The model under review builds one solid part; all positions refer to its coordinate system, in mm. Face numbers are marked on the shaded views. Give positions to 0.01 mm unless a question says otherwise; leave off trailing zeros. Order: outer loops, then holes, each group sorted by start corner. A loop starts at its lowest first (then second) coordinate and runs counter-clockwise, first axis right, second up. Notation, with made-up numbers: (76, 69.25) - (132, 69.25) arc R19 cw to (132, 91.25) - close; hole circle Ø7 at (-3.75, 0.5). An arc over 180 degrees is marked (long way). Use CSV: the item, a comma, the result in double quotes. Start each with the question number.
1. Take a section at A-A, the plane z = -17.68. State the section outline as (x, y) points.
2. Take a section at B-B, the plane x = 0. State the section outline as (y, z) points (3 decimals), then the cut area to 3 significant figures.
3. For pin 1 (3 mm diameter, centred on x = 40.5, y = 1, fed in from -Z), flat-tipped, find the tip position at first contact; note if it passes through.
4. To check wall thickness, follow line 1 (X direction, y = 1.6, z = -35.36) (3 decimals); line 2 (Z direction, x = 0, y = 2.2) (3 decimals); line 3 (Z direction, x = 17.68, y = 2.3). State the ranges of each line that lie inside material, in increasing order. Write a range as [from, to].
5. Take a section at C-C, the plane y = 2.95. State the section outline as (x, z) points (3 decimals), then the cut area to 3 significant figures.
6. Draft analysis for pull direction X (two halves, no side actions). For the marked faces 1, 2 and 3, state which applies: released by +X, released by -X, zero draft, split by the parting line, or undercut.
7. Take a section at D-D, the plane z = -35.36. State the section outline as (x, y) points (3 decimals), then the cut area to 3 significant figures.
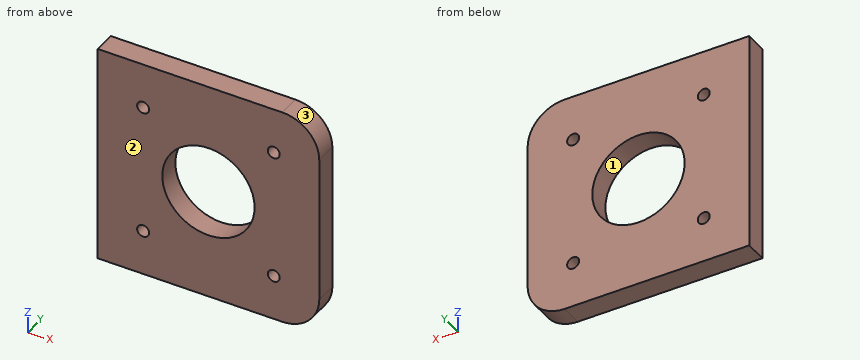
```python
from build123d import *

# Parameters (mm, degrees)
SKETCH1_W           = 60
SKETCH1_H           = 60
SKETCH1_R           = 1.625
SKETCH1_R_2         = 12.5
BOSS_EXTRUDE1_DEPTH = 6
FILLET1_R           = 10


with BuildPart() as part:
    # Sketch1 → Boss-Extrude1 (new body)
    with BuildSketch(Plane(origin=(0, 0, 0), x_dir=(1, 0, 0), z_dir=(0, 1, 0))):
        with Locations((17.68, 17.68)):
            Rectangle(SKETCH1_W, SKETCH1_H)
        with Locations((0, 35.36)):
            Circle(SKETCH1_R, mode=Mode.SUBTRACT)
        with Locations((35.36, 35.36)):
            Circle(SKETCH1_R, mode=Mode.SUBTRACT)
        with Locations((35.36, 0)):
            Circle(SKETCH1_R, mode=Mode.SUBTRACT)
        Circle(SKETCH1_R, mode=Mode.SUBTRACT)
        with Locations((17.68, 17.68)):
            Circle(SKETCH1_R_2, mode=Mode.SUBTRACT)
    extrude(amount=BOSS_EXTRUDE1_DEPTH)

    # Fillet1
    fillet1_edges = [part.edges().sort_by_distance(p)[0] for p in [
        (47.68, 3, -47.68),
        (47.68, 3, 12.32),
    ]]
    fillet(fillet1_edges, radius=FILLET1_R)


solid = part.part
```
Determined:
1,outline,"(-12.32, 0) - (5.18, 0) - (5.18, 6) - (-12.32, 6) - close; (30.18, 0) - (47.68, 0) - (47.68, 6) - (30.18, 6) - close"
2,outline,"(0, -47.68) - (6, -47.68) - (6, -36.985) - (0, -36.985) - close; (0, -33.735) - (6, -33.735) - (6, -1.625) - (0, -1.625) - close; (0, 1.625) - (6, 1.625) - (6, 12.32) - (0, 12.32) - close"
2,area,"321 mm²"
3,pin 1,"stops at z = -47.59"
4,line 1,"x = [-12.32, -1.625], [1.625, 33.735], [36.985, 47.68]"
4,line 2,"z = [-47.68, -36.985], [-33.735, -1.625], [1.625, 12.32]"
4,line 3,"z = [-47.68, -30.18], [-5.18, 12.32]"
5,outline,"(-12.32, -47.68) - (37.68, -47.68) arc R10 ccw to (47.68, -37.68) - (47.68, 2.32) arc R10 ccw to (37.68, 12.32) - (-12.32, 12.32) - close; hole circle Ø3.25 at (0, -35.36); hole circle Ø3.25 at (0, 0); hole circle Ø25 at (17.68, -17.68); hole circle Ø3.25 at (35.36, -35.36); hole circle Ø3.25 at (35.36, 0)"
5,area,"3,030 mm²"
6,face 1,"undercut"
6,face 2,"zero draft"
6,face 3,"released by +X"
7,outline,"(-12.32, 0) - (-1.625, 0) - (-1.625, 6) - (-12.32, 6) - close; (1.625, 0) - (33.735, 0) - (33.735, 6) - (1.625, 6) - close; (36.985, 0) - (47.68, 0) - (47.68, 6) - (36.985, 6) - close"
7,area,"321 mm²"
